Autodesk Inventor part; units mm, degrees
ref_plane "YZ Plane" through (0, 0, 0) normal (1, 0, 0) x (0, 1, 0)
ref_plane "XZ Plane" through (0, 0, 0) normal (0, 1, 0) x (-1, 0, 0)
ref_plane "XY Plane" through (0, 0, 0) normal (0, 0, 1) x (1, 0, 0)
sketch "Sketch1" plane through (0, 0, 0) normal (0, 1, 0) x (-1, 0, 0)
  line L0 (0, 30) -> (0, -30) construction
  line L1 (-2.5, 30) -> (-2.5, -30)
  line L2 (2.5, -30) -> (2.5, 30)
  arc A0 (2.5, 30) -> (-2.5, 30) centre (0, 30) ccw
  arc A1 (-2.5, -30) -> (2.5, -30) centre (0, -30) ccw
  point P0 (0, 0)
  point P1 (0, 0)
  dimension "d0" = 60
  dimension "d1" = 5
extrude "Extrusion1" add sketch "Sketch1" along normal blind 3.75
sketch "Sketch2" plane through (0, 3.75, 0) normal (0, 1, 0) x (1, 0, 0)
  arc A0 (2.5, 30) -> (-2.5, 30) centre (0, 30) ccw
  line L0 (-2.5, 30) -> (-2.5, -30)
  arc A1 (-2.5, -30) -> (2.5, -30) centre (0, -30) ccw
  line L1 (2.5, -30) -> (2.5, 30)
  point P0 (0, 0)
hole "Hole1" at (0, 3.75, 30) at (0, 3.75, -30) direction (0, -1, 0) diameter 3.4 end through all
sketch "Sketch3" plane through (0, 3.75, 0) normal (0, 1, 0) x (1, 0, 0)
  line L0 (2.5, 5) -> (2.5, -5) construction
  line L1 (2.5, -30) -> (2.5, 30)
  line L2 (1, 5) -> (1, -5)
  line L3 (4, -5) -> (4, 5)
  arc A0 (4, 5) -> (1, 5) centre (2.5, 5) ccw
  arc A1 (1, -5) -> (4, -5) centre (2.5, -5) ccw
  point P0 (0, 0)
  point P1 (2.5, 0)
  point P2 (2.5, -6.5)
  point P3 (2.5, 6.5)
  dimension "d11" = 5
  dimension "d12" = 3
extrude "Extrusion2" cut sketch "Sketch3" against normal through all contours A1 L2 A0 L1
properties part number "MainLink"
Check sheet for the modelled part. Datum: model origin and axes. Units: mm. A direction names the side the tool comes from. Round coordinates to 2 decimals unless told otherwise and drop trailing zeros. Loops run counter-clockwise (first coordinate to the right, second up) from the corner with the lowest first, then second, coordinate; pieces in that order, holes last. Notation, with made-up numbers: M 14.5,43.25 L 38.5,43.25 A36 ccw 38.5,80.25 Z; hole C 12,-2.5 d1. An arc over 180 degrees is marked long. One line per question, with ' | ' between items. Start each with the question number.
Item 1: Section check A-A (y = 1.05). Record the boundary of the cut face in (x, z), and give its area (3 significant figures).
Item 2: Set-up check for faces 1 (the face through (-0.1, 1.8, -32.5)), 2 (the face through (1, 2, 0)): record each of +Z, -Z, +X, -X, +Y, -Y from which the full face is reachable in a straight line by a thin tool's end or side.
Item 3: Section check B-B (x = -0.9). Record the boundary of the cut face in (y, z), and give its area (3 significant figures).
Item 4: Release check for a two-part mould opening along Z. For faces 3 (the face through (0.1, 1.8, 32.5)), 4 (the face through (1.43, 1.9, 6.05)), 5 (the face through (0, 3.75, 0)) record: released by +Z, released by -Z, zero draft, split by the parting line, or undercut.
Item 5: Scan lines: probe 1 along Z at (x, y) = (0.05, 2.05); probe 2 along X at (y, z) = (1.4, -30); probe 3 along Z at (x, y) = (0.7, 1.1). Record each from-to range of solid material in increasing order.
Worked out:
1) outline: M -2.5,-30 A2.5 ccw 2.5,-30 L 2.5,-6.5 A1.5 cw 1,-5 L 1,5 A1.5 cw 2.5,6.5 L 2.5,30 A2.5 ccw -2.5,30 Z; hole C 0,-30 d3.4; hole C 0,30 d3.4 | area: 283 mm^2
2) face 1: -Z, +Y, -Y | face 2: +X, +Y, -Y
3) outline: M 0,-32.33 L 3.75,-32.33 L 3.75,-31.44 L 0,-31.44 Z; M 0,-28.56 L 3.75,-28.56 L 3.75,28.56 L 0,28.56 Z; M 0,31.44 L 3.75,31.44 L 3.75,32.33 L 0,32.33 Z | area: 221 mm^2
4) face 3: released by +Z | face 4: undercut | face 5: zero draft
5) probe 1: -32.5 to -31.7, -28.3 to 28.3, 31.7 to 32.5 | probe 2: -2.5 to -1.7, 1.7 to 2.5 | probe 3: -32.4 to -31.55, -28.45 to 28.45, 31.55 to 32.4
